Here's how the part is built. I have some questions about the finished solid (model axes, mm). A direction names the side the tool comes from. Give positions to 0.01 mm unless a question says otherwise; leave off trailing zeros. Loops run counter-clockwise (first coordinate to the right, second up) from the corner with the lowest first, then second, coordinate; pieces in that order, holes last.
Q1. We'd pull the mould along Y, two halves only. Please class faces 1 (the face through (0, 14, 3.2)), 2 (the face through (10, 10, 5)), 3 (the face through (0.14, -1.195, 5.315)): +Y half, -Y half, draft (parallel to the pull), parting line (faces both ways), or undercut.
Q2. Will these pins go through, and if not, where does the flat tip stop? P1, Ø6, axis at x = -1.5, y = 2, coming from the +Z side; P2, Ø2, axis at x = -0.5, y = 5, coming from the +Z side; P3, Ø1, axis at x = 5.5, z = 9, coming from the -Y side; P4, Ø1, axis at y = 15, z = 4.5, coming from the -X side.
Q3. If we section it at A-A (x = 5): Please give me the cut outline in (y, z) (3 decimals).
Q4. If we section it at C-C (y = 19): Please give me the cut outline in (x, z), plus the area to 3 significant figures.
Q5. I need wall thicknesses on line 1 (Z direction, x = -2.75, y = 12); line 2 (Z direction, x = -4.25, y = 10.5); line 3 (Z direction, x = -4.5, y = 17.25). Which ranges of each line are inside material? Lowest first, please.
Q6. If we section it at B-B (z = 2.5): Please give me the cut outline in (x, y), plus the area to 3 significant figures.
Q7. If we section it at D-D (x = 0.75): Please give me the cut outline in (y, z) (3 decimals).
Q8. For faces 4 (the face through (0.14, 11.67, 12.19)), 5 (the face through (0.14, -1.318, 2.283)), 6 (the face through (0.14, 0.98, 4.7)), which set-ups out of +Z, -Z, +X, -X, +Y, -Y let a thin tool reach every point of the face, with its end or its side?
from build123d import *

# Parameters (mm, degrees)
F1_DEPTH = 10
F3_DEPTH = 3.2


with BuildPart() as f1:
    # F0 (on Right) → F1 (new body, symmetric)
    with BuildSketch(Plane.YZ):
        with BuildLine():
            Line((-2.6, 4.5033320997), (0, 0))
            Line((0, 0), (20, 0))
            Line((20, 0), (20, 3.2))
            ThreePointArc((20, 3.2), (19, 4.2), (18, 3.2))
            Line((18, 3.2), (9.8790542573, 3.2))
            ThreePointArc((9.8790542573, 3.2), (9.5728680395, 3.0952847075), (9.394931339, 2.825))
            ThreePointArc((9.394931339, 2.825), (6.4936738448, 2.8117714323), (9.0128508216, 4.2509439038))
            ThreePointArc((9.0128508216, 4.2509439038), (9.3020908782, 4.1058388311), (9.6196135673, 4.1682458366))
            Line((9.6196135673, 4.1682458366), (17.4008928334, 8.6607695155))
            Line((17.4008928334, 8.6607695155), (13.6008928334, 15.2425625842))
            Line((13.6008928334, 15.2425625842), (10.8296115413, 13.6425625842))
            Line((10.8296115413, 13.6425625842), (12.5296115413, 10.6980762114))
            ThreePointArc((12.5296115413, 10.6980762114), (12.6295119638, 9.9392571663), (12.1635861375, 9.3320508076))
            Line((12.1635861375, 9.3320508076), (1.7712812921, 3.3320508076))
            Line((1.7712812921, 3.3320508076), (0.1712812921, 6.1033320997))
            Line((0.1712812921, 6.1033320997), (-2.6, 4.5033320997))
        make_face()
    extrude(amount=F1_DEPTH, both=True)

    # F2 (on face) → F3 (cut, through all)
    with BuildSketch(Plane(origin=(0, 14.0296115413, 8.1), x_dir=(1, 0, 0), z_dir=(0, -0.8660254038, -0.5))):
        with BuildLine():
            Line((4.3634848459, 6.4), (-4.3634848459, 6.4))
            ThreePointArc((-4.3634848459, 6.4), (0, 5), (4.3634848459, 6.4))
        make_face()
    extrude(amount=-F3_DEPTH, mode=Mode.SUBTRACT)


solid = f1.part
Check sheet entries:
1. face 1: undercut
1. face 2: draft
1. face 3: -Y half
2. P1: stops at z = 6.1
2. P2: stops at z = 5.77
2. P3: stops at y = 10.72
2. P4: passes through
3. outline: (-2.6, 4.503) - (0, 0) - (20, 0) - (20, 3.2) arc R1 ccw to (18, 3.2) - (9.879, 3.2) arc R0.5 ccw to (9.395, 2.825) arc R1.5 cw (long way) to (9.013, 4.251) arc R0.5 ccw to (9.62, 4.168) - (17.401, 8.661) - (13.601, 15.243) - (10.83, 13.643) - (12.53, 10.698) arc R1 cw to (12.164, 9.332) - (1.771, 3.332) - (0.171, 6.103) - close
4. outline: (-10, 0) - (10, 0) - (10, 4.2) - (-10, 4.2) - close
4. area: 84.0 mm2
5. line 1: z = 0 to 3.2, 5.54 to 9.24, 11.62 to 13.3
5. line 2: z = 0 to 3.2, 4.68 to 8.37
5. line 3: z = 0 to 3.2, 8.57 to 8.92
6. outline: (-10, -1.44) - (10, -1.44) - (10, 6.62) - (-10, 6.62) - close; (-10, 9.27) - (10, 9.27) - (10, 20) - (-10, 20) - close
6. area: 376 mm2
7. outline: (-2.6, 4.503) - (0, 0) - (20, 0) - (20, 3.2) arc R1 ccw to (18, 3.2) - (9.879, 3.2) arc R0.5 ccw to (9.395, 2.825) arc R1.5 cw (long way) to (9.013, 4.251) arc R0.5 ccw to (9.62, 4.168) - (17.401, 8.661) - (14.282, 14.063) - (11.511, 12.463) - (12.53, 10.698) arc R1 cw to (12.164, 9.332) - (1.771, 3.332) - (0.171, 6.103) - close
8. face 4: +X, -X, -Y
8. face 5: -Z, +X, -X, -Y
8. face 6: +Z, +X, -X
